Source: three-view drawing plus pictorial views. Frame: mm from the lowest corner of the part. Give positions to 0.01 mm unless a question says otherwise; leave off trailing zeros. Loops run counter-clockwise (first coordinate to the right, second up) from the corner with the lowest first, then second, coordinate; pieces in that order, holes last. Notation, with made-up numbers: (59.25, -30.75) - (112.25, -30.75) arc R28 cw to (112.25, 0.25) - close; hole circle Ø11 at (27.25, -5). An arc over 180 degrees is marked (long way). Write each question's results on one line, items separated by ' | '. Start each with the question number.
(1) Contact query for flat-ended pins moving along their axis: pin 1 (1.2 mm diameter, centred on y = 16.5, z = 7.5, fed in from -X); pin 2 (5 mm diameter, centred on x = 24.75, y = 16.75, fed in from +Z); pin 3 (8 mm diameter, centred on x = 49, z = 22, fed in from -Y); pin 4 (3 mm diameter, centred on y = 16.75, z = 17.5, fed in from +X). Output: stop coordinate, or through.
(2) Cut plane C-C on y = 16.75. Return the cut outline in (x, z).
(3) Cut plane A-A on z = 7.5. Give the number of separate pieces and of enclosed holes in the cut face, then the cut area to 3 significant figures.
(4) Material intervals for line 1 along Y through (x, z) = (24.75, 7.5); line 2 along Z through (x, y) = (9.5, 17.5) (1 decimal); line 3 along X through (y, z) = (18, 12.5) (1 decimal), sorted ascending. Write a range as [from, to].
(5) Cut plane B-B on x = 24.75. Return the cut outline in (y, z).
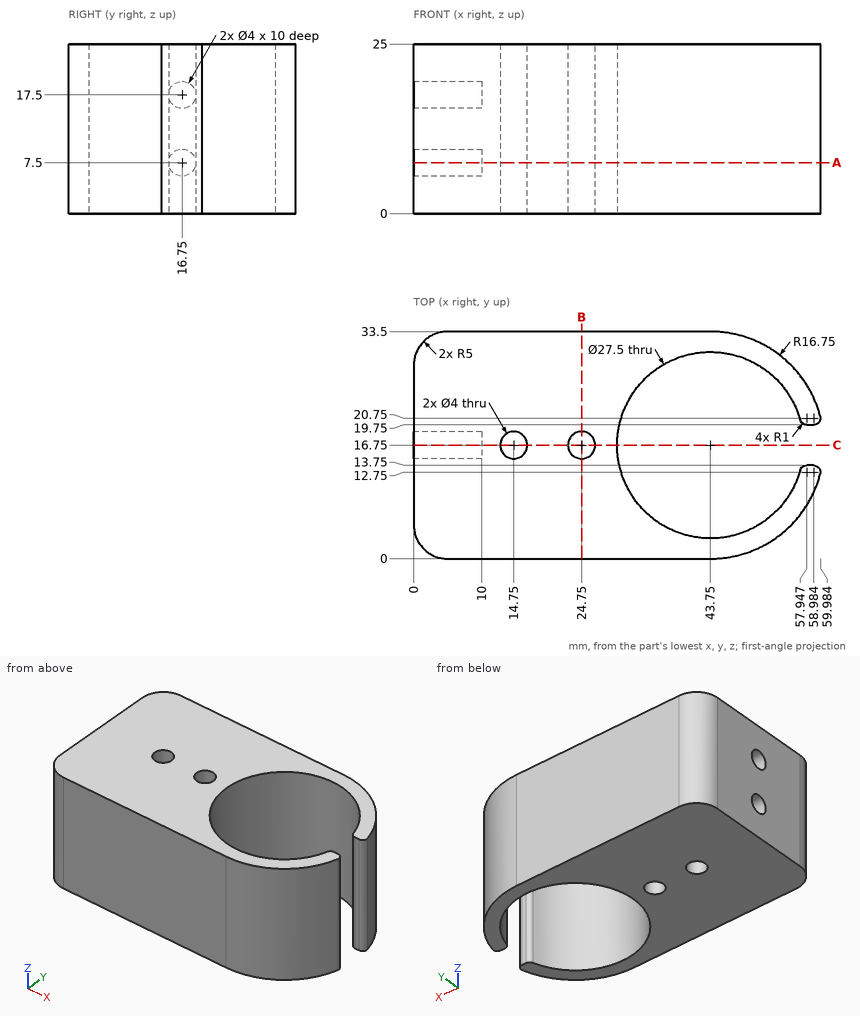
Ans:
1) pin 1: x = 10 | pin 2: z = 25 | pin 3: y = 0.05 | pin 4: x = 30.08
2) outline: (0, 0) - (12.75, 0) - (12.75, 25) - (0, 25) - (0, 19.5) - (10, 19.5) - (10, 15.5) - (0, 15.5) - (0, 9.5) - (10, 9.5) - (10, 5.5) - (0, 5.5) - close; (16.75, 0) - (22.75, 0) - (22.75, 25) - (16.75, 25) - close; (26.75, 0) - (30, 0) - (30, 25) - (26.75, 25) - close
3) separate pieces: 1 | enclosed holes: 2 | area: 1,220 mm^2
4) line 1: [0, 14.75], [18.75, 33.5] | line 2: [0, 5.6], [9.4, 15.6], [19.4, 25] | line 3: [0, 13.2], [16.3, 23.2], [26.3, 30.1]
5) outline: (0, 0) - (14.75, 0) - (14.75, 25) - (0, 25) - close; (18.75, 0) - (33.5, 0) - (33.5, 25) - (18.75, 25) - close
